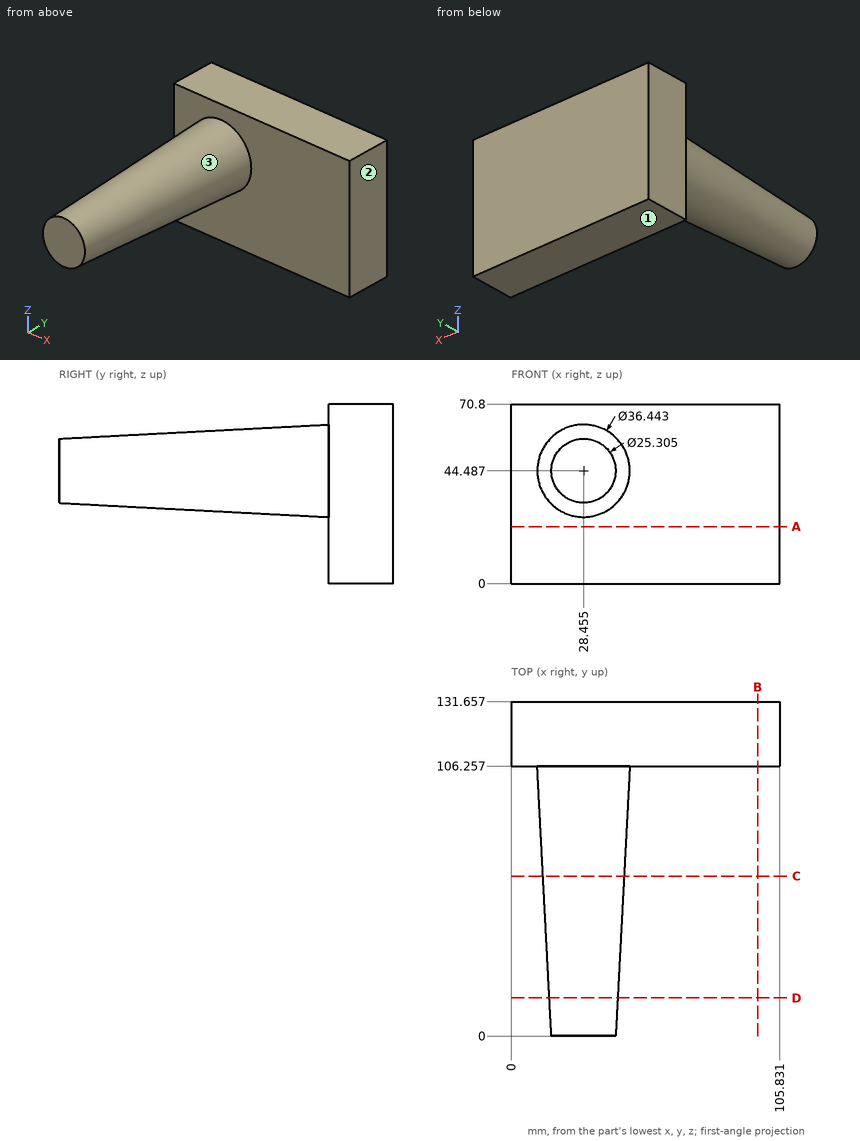
Print and shaded views of the part. All mm, measured from the part's lowest x, y and z. Coordinates: 2 decimals unless noted, no trailing zeros. Order: outer loops, then holes, each group sorted by start corner. A loop starts at its lowest first (then second) coordinate and runs counter-clockwise, first axis right, second up. Notation, with made-up numbers: M -10.5,-26.75 L 20.5,-26.75 A18 ccw 20.5,1.25 Z; hole C 86.25,48.25 d8. An arc over 180 degrees is marked long. Answer as CSV lines item,"result".
1) Drill centre lines: L1, parallel to Y at x = 53, z = 10.5; L2, parallel to X at y = 75, z = 53.5 (1 decimal); L3, parallel to X at y = 31.5, z = 42. Where is each one in solid material? Low to high. Write a range as from..to.
Verdict:
L1,"106.26..131.66"
L2,"14.5..42.4"
L3,"14.37..42.54"
2) Cut at B-B (x = 97). List the corners of the cut face in (y, z).
Verdict:
outline,"M 106.26,0 L 131.66,0 L 131.66,70.8 L 106.26,70.8 Z"
3) Cut at A-A (z = 22.5). List the corners of the cut face in (x, y), then the cut area to 3 significant figures.
Verdict:
outline,"M 0,106.26 L 105.83,106.26 L 105.83,131.66 L 0,131.66 Z"
area,"2,690 mm2"
4) Mould opens along Z. For the marked faces 1, 2 and 3 say: released by +Z, released by -Z, zero draft, split by the parting line, or undercut.
Verdict:
face 1,"released by -Z"
face 2,"zero draft"
face 3,"split by the parting line"
5) Cut at C-C (y = 63). List the corners of the cut face in (x, z) (1 decimal).
Verdict:
outline,"C 28.5,44.5 d31.9"
6) Flat gauge pins, fed straight in: P1, Ø4, axis at x = 92, z = 12.5, coming from the -Y side; P2, Ø8, axis at y = 21.5, z = 54.5, coming from the -X side. Where does each tip first touch, or does it go through?
Verdict:
P1,"y = 106.26"
P2,"x = 16.04"
7) Cut at D-D (y = 15). List the corners of the cut face in (x, z) (1 decimal).
Verdict:
outline,"C 28.5,44.5 d26.9"
